Check sheet for the drawn part. Datum: minimum x, y, z corner. Units: mm. A direction names the side the tool comes from. Round coordinates to 2 decimals unless told otherwise and drop trailing zeros. Loops run counter-clockwise (first coordinate to the right, second up) from the corner with the lowest first, then second, coordinate; pieces in that order, holes last.
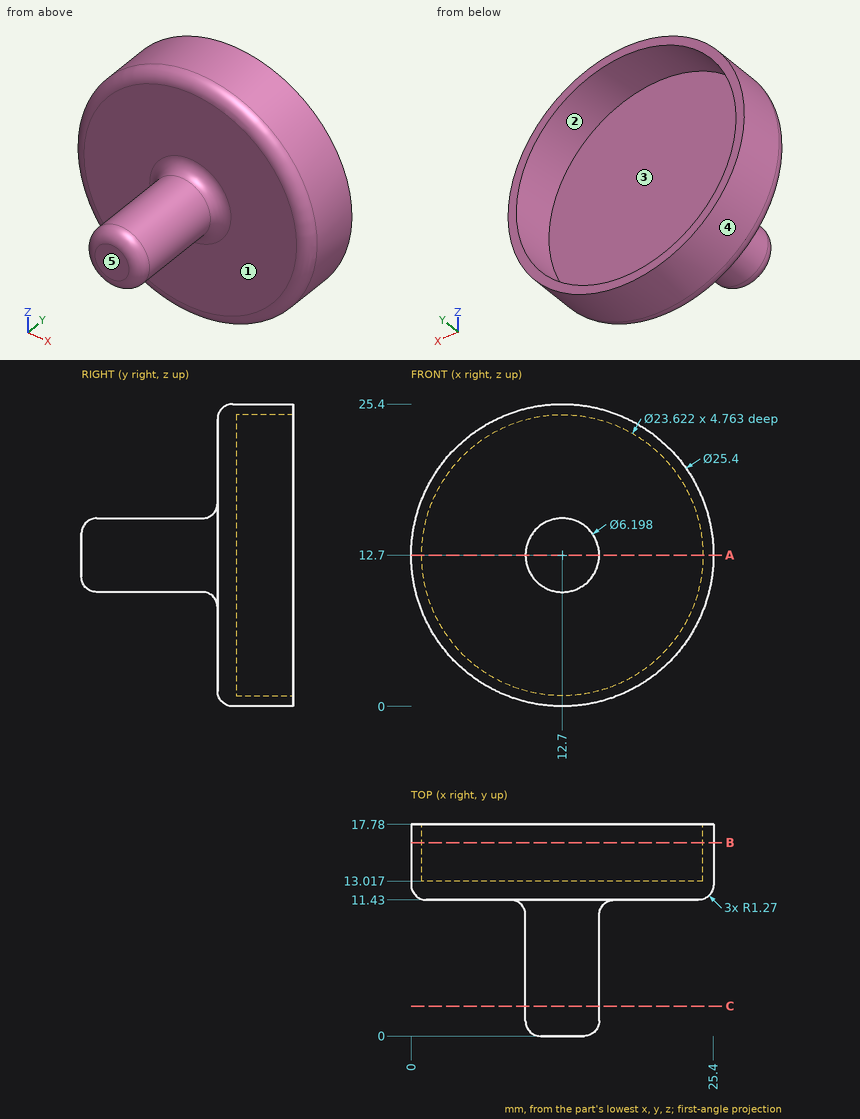
1) Access from +Z, -Z, +X, -X, +Y, -Y to the whole of each face (thin tool, end or side, straight path). Record for the marked faces 1 and 2.
Report:
face 1: -Y
face 2: +Y
2) Scan lines: line 1 along X through (y, z) = (16.5, 12.7); line 2 along Y through (x, z) = (12.5, 20.5); line 3 along X through (y, z) = (14.25, 21.25). Record each from-to range of solid material in increasing order.
Report:
line 1: x = 0 to 0.89, 24.51 to 25.4
line 2: y = 11.43 to 13.02
line 3: x = 3.31 to 4.55, 20.85 to 22.09
3) Sectioned sample at A-A, the plane z = 12.7. Record the cut outline in (x, y).
Report:
outline: (0, 12.7) arc R1.27 ccw to (1.27, 11.43) - (8.33, 11.43) arc R1.27 cw to (9.6, 10.16) - (9.6, 1.27) arc R1.27 ccw to (10.87, 0) - (14.53, 0) arc R1.27 ccw to (15.8, 1.27) - (15.8, 10.16) arc R1.27 cw to (17.07, 11.43) - (24.13, 11.43) arc R1.27 ccw to (25.4, 12.7) - (25.4, 17.78) - (24.51, 17.78) - (24.51, 13.02) - (0.89, 13.02) - (0.89, 17.78) - (0, 17.78) - close
4) Sectioned sample at B-B, the plane y = 16.25. Record the cut outline in (x, z).
Report:
outline: circle Ø25.4 at (12.7, 12.7); hole circle Ø23.62 at (12.7, 12.7)
5) Mould release check, pull along X, two halves, no side actions. Record for the marked faces 3, 4 and 5: +X half, -X half, draft (parallel to the pull), parting line (faces both ways), or undercut.
Report:
face 3: undercut
face 4: parting line
face 5: draft
6) Sectioned sample at C-C, the plane y = 2.5. Record the cut outline in (x, z).
Report:
outline: circle Ø6.2 at (12.7, 12.7)
7) Gauge pin test, flat ends, axial feed: pin 1 (5 mm diameter, centred on x = 12.5, y = 6, fed in from -Z); pin 2 (1 mm diameter, centred on x = 22.5, z = 4.5, fed in from -Y) (1 decimal); pin 3 (7 mm diameter, centred on x = 15.5, z = 9, fed in from +Y). Record the tip position at first contact, or that the pin passes through.
Report:
pin 1: stops at z = 9.6
pin 2: stops at y = 11.8
pin 3: stops at y = 13.02
